Read the model definition and answer for the solid it produces. Units are mm, in the model's axes. Give positions to 0.01 mm unless a question says otherwise; leave off trailing zeros. Loops run counter-clockwise (first coordinate to the right, second up) from the corner with the lowest first, then second, coordinate; pieces in that order, holes last. Notation, with made-up numbers: (2, 5) - (37, 5) arc R33 ccw to (37, 43) - close; hole circle Ø7 at (9.25, -36.75). An arc over 180 degrees is marked (long way). Put each result on its own line as item: value. Start each with the question number.
1. A cutting plane is placed at A-A, the plane y = 0. Determine the outline of the cut face in (x, z).
2. For a pull along Y with two mould halves and no side action, classify faces 1 (the cylindrical face through (-1.216, 1.115, -0.986)), 2 (the flat face through (0, -5, -1)), 3 (the flat face through (-35, 0, -1)) as released by +Y, released by -Y, zero draft, split by the parting line, or undercut.
3. A cutting plane is placed at B-B, the plane x = 0. Determine the outline of the cut face in (y, z).
4. Consider L1, parallel to Y at x = 0, z = -1.5; L2, parallel to X at y = -1.5, z = -1.05; L3, parallel to X at y = -0.5, z = -0.15. Determine where each line is inside the solid, lowest interval first. Write a range as from..to.
```python
from build123d import *

# Parameters (mm, degrees)
ESBO_O1_W                                      = 70
ESBO_O1_H                                      = 10
FLANGE_BASE1_DEPTH                             = 2
BROCA_DE_ROSQUEAR_DE_CANO_PARA_TARRAXA_D_D     = 3.3
BROCA_DE_ROSQUEAR_DE_CANO_PARA_TARRAXA_D_DEPTH = 4
BROCA_DE_ROSQUEAR_DE_CANO_PARA_TARRAXA_D_TIP   = 0.991420021


# Sheet-metal steps are written as plain solids
with BuildPart() as part:
    # Esboço1 → Flange-base1 (new body)
    with BuildSketch(Plane.XY):
        Rectangle(ESBO_O1_W, ESBO_O1_H)
    extrude(amount=-FLANGE_BASE1_DEPTH)

    # Broca de rosquear de cano para tarraxa de 1/81
    with Locations(Plane(origin=(0, 0, -2), x_dir=(-1, 0, 0), z_dir=(0, 0, -1))):
        with Locations((0, 0)):
            Hole(BROCA_DE_ROSQUEAR_DE_CANO_PARA_TARRAXA_D_D / 2, depth=BROCA_DE_ROSQUEAR_DE_CANO_PARA_TARRAXA_D_DEPTH)
            with Locations((0, 0, -(BROCA_DE_ROSQUEAR_DE_CANO_PARA_TARRAXA_D_DEPTH + BROCA_DE_ROSQUEAR_DE_CANO_PARA_TARRAXA_D_TIP / 2))):  # 118° drill point
                Cone(0, BROCA_DE_ROSQUEAR_DE_CANO_PARA_TARRAXA_D_D / 2, BROCA_DE_ROSQUEAR_DE_CANO_PARA_TARRAXA_D_TIP, mode=Mode.SUBTRACT)


solid = part.part
```
Return value:
1. outline: (-35, -2) - (-1.65, -2) - (-1.65, 0) - (-35, 0) - close; (1.65, -2) - (35, -2) - (35, 0) - (1.65, 0) - close
2. face 1: undercut
2. face 2: released by -Y
2. face 3: zero draft
3. outline: (-5, -2) - (-1.65, -2) - (-1.65, 0) - (-5, 0) - close; (1.65, -2) - (5, -2) - (5, 0) - (1.65, 0) - close
4. L1: y = -5..-1.65, 1.65..5
4. L2: x = -35..-0.69, 0.69..35
4. L3: x = -35..-1.57, 1.57..35
